from build123d import *

# Parameters (mm, degrees)
SKETCH1_W           = 35.56
SKETCH1_H           = 25.4
BOSS_EXTRUDE1_DEPTH = 2.54
SKETCH2_W           = 2.54
SKETCH2_H           = 2.54
BOSS_EXTRUDE2_DEPTH = 2.54
SKETCH4_W           = 2.54
SKETCH4_H           = 2.54
BOSS_EXTRUDE4_DEPTH = 1.27
SKETCH5_W           = 2.54
SKETCH5_H           = 2.54
BOSS_EXTRUDE5_DEPTH = 17.78


with BuildPart() as part:
    # Sketch1 → Boss-Extrude1 (new body)
    with BuildSketch(Plane.XY):
        with Locations((-17.78, 12.7)):
            Rectangle(SKETCH1_W, SKETCH1_H)
    extrude(amount=BOSS_EXTRUDE1_DEPTH)

    # Sketch2 → Boss-Extrude2 (add)
    with BuildSketch(Plane.XY.offset(2.54)):
        with Locations((-34.29, 24.13)):
            Rectangle(SKETCH2_W, SKETCH2_H)
        with Locations((-1.27, 24.13)):
            Rectangle(SKETCH2_W, SKETCH2_H)
        with Locations((-1.27, 1.27)):
            Rectangle(SKETCH2_W, SKETCH2_H)
        with Locations((-34.29, 1.27)):
            Rectangle(SKETCH2_W, SKETCH2_H)
    boss_extrude2 = extrude(amount=BOSS_EXTRUDE2_DEPTH)

    # Mirror1: Boss-Extrude2 across plane
    add(boss_extrude2.mirror(Plane.XY.offset(1.27)))

    # Sketch4 → Boss-Extrude4 (add)
    with BuildSketch(Plane.ZY.offset(35.56)):
        with Locations((3.81, 24.13)):
            Rectangle(SKETCH4_W, SKETCH4_H)
        with Locations((-1.27, 24.13)):
            Rectangle(SKETCH4_W, SKETCH4_H)
        with Locations((3.81, 1.27)):
            Rectangle(SKETCH4_W, SKETCH4_H)
        with Locations((-1.27, 1.27)):
            Rectangle(SKETCH4_W, SKETCH4_H)
    boss_extrude4 = extrude(amount=BOSS_EXTRUDE4_DEPTH)

    # Mirror2: Boss-Extrude4 across plane
    add(boss_extrude4.mirror(Plane.ZY.offset(17.78)))

    # Sketch5 → Boss-Extrude5 (add)
    with BuildSketch(Plane(origin=(0, 25.4, 0), x_dir=(1, 0, 0), z_dir=(0, 1, 0))):
        with Locations((-34.29, -1.27)):
            Rectangle(SKETCH5_W, SKETCH5_H)
        with Locations((-1.27, -1.27)):
            Rectangle(SKETCH5_W, SKETCH5_H)
    extrude(amount=BOSS_EXTRUDE5_DEPTH)


solid = part.part
For this review, take the finished solid that the model builds, in its own axes (mm). A direction names the side the tool comes from. Give positions to 0.01 mm unless a question says otherwise; leave off trailing zeros. Order: outer loops, then holes, each group sorted by start corner. A loop starts at its lowest first (then second) coordinate and runs counter-clockwise, first axis right, second up. Notation, with made-up numbers: (69.25, 21) - (79.25, 21) arc R10 ccw to (79.25, 37) - close; hole circle Ø3 at (6.5, 65.5). An arc over 180 degrees is marked (long way). Answer as a JSON object with one key per item and string values. Group by question number.
Item 1: Take a section at D-D on y = 23.5. Give the boundary of the cut face in (x, z).
Item 2: Wall thickness on line 1 along X through (y, z) = (35.5, 0.75); line 2 along X through (y, z) = (23, 3.25); line 3 along X through (y, z) = (3, 2.25): over which ranges is each line inside the solid? List them lowest first.
Item 3: Clearance check with flat-ended pins moving along their axes: pin 1 Ø6 at (x, y) = (-17, 26) entering from -Z; pin 2 Ø1.3 at (x, z) = (-35, -1) entering from +Y; pin 3 Ø2 at (y, z) = (35, 1) entering from +X; pin 4 Ø2 at (x, y) = (-31.5, 27.5) entering from -Z. State where each tip first meets the part, or that it passes through.
Item 4: Take a section at C-C on z = 1.75. Give the boundary of the cut face in (x, y), and give its area (3 significant figures).
Item 5: Take a section at A-A on z = -2. Give the boundary of the cut face in (x, y), and give its area (3 significant figures).
Item 6: Take a section at B-B on y = 30. Give the boundary of the cut face in (x, z).
Item 7: Machinability: for faces 5 (the flat face through (-33.02, 24, -1)), 6 (the flat face through (-33.02, 34, 1)), 7 (the flat face through (-1, 1, 5.08)), 8 (the flat face through (-1, 34, 0)), 9 (the flat face through (-1, 25.4, 4)), which of the approach directions +Z, -Z, +X, -X, +Y, -Y give a long, thin tool a straight path to every point of the face, cutting with its end or side? Answer none if there is none.
Item 8: Draft analysis for pull direction Z (two halves, no side actions). For faces 1 (the flat face through (-36, 24, 0)), 2 (the flat face through (-1, 24, -2.54)), 3 (the flat face through (-36.83, 24, 4)), 4 (the flat face through (-36, 1, 0)), state which applies: pulls with the +Z half, pulls with the -Z half, needs draft (parallel to the pull), parting line crosses it, or undercut.
Reported:
{
 "1": {"outline": "(-36.83, -2.54) - (-33.02, -2.54) - (-33.02, 0) - (-2.54, 0) - (-2.54, -2.54) - (1.27, -2.54) - (1.27, 0) - (0, 0) - (0, 2.54) - (1.27, 2.54) - (1.27, 5.08) - (-2.54, 5.08) - (-2.54, 2.54) - (-33.02, 2.54) - (-33.02, 5.08) - (-36.83, 5.08) - (-36.83, 2.54) - (-35.56, 2.54) - (-35.56, 0) - (-36.83, 0) - close"},
 "2": {"line 1": "-35.56 to -33.02, -2.54 to 0", "line 2": "-36.83 to -33.02, -2.54 to 1.27", "line 3": "-35.56 to 0"},
 "3": {"pin 1": "z = 0", "pin 2": "y = 25.4", "pin 3": "x = 0", "pin 4": "through"},
 "4": {"outline": "(-35.56, 0) - (0, 0) - (0, 43.18) - (-2.54, 43.18) - (-2.54, 25.4) - (-33.02, 25.4) - (-33.02, 43.18) - (-35.56, 43.18) - close", "area": "994 mm^2"},
 "5": {"outline": "(-36.83, 0) - (-33.02, 0) - (-33.02, 2.54) - (-36.83, 2.54) - close; (-36.83, 22.86) - (-33.02, 22.86) - (-33.02, 25.4) - (-36.83, 25.4) - close; (-2.54, 0) - (1.27, 0) - (1.27, 2.54) - (-2.54, 2.54) - close; (-2.54, 22.86) - (1.27, 22.86) - (1.27, 25.4) - (-2.54, 25.4) - close", "area": "38.7 mm^2"},
 "6": {"outline": "(-35.56, 0) - (-33.02, 0) - (-33.02, 2.54) - (-35.56, 2.54) - close; (-2.54, 0) - (0, 0) - (0, 2.54) - (-2.54, 2.54) - close"},
 "7": {"face 5": "-Z, +Y, -Y", "face 6": "+Z, -Z, +Y", "face 7": "+Z, +X, -X, +Y, -Y", "face 8": "-Z, +X, -X, +Y", "face 9": "+Z, +X, -X, +Y"},
 "8": {"face 1": "undercut", "face 2": "pulls with the -Z half", "face 3": "needs draft", "face 4": "undercut"}
}
